Geometry: see drawing. Coordinates: mm, zero at the bounding-box minimum. Coordinates: 2 decimals unless noted, no trailing zeros. Loops run counter-clockwise (first coordinate to the right, second up) from the corner with the lowest first, then second, coordinate; pieces in that order, holes last. Notation, with made-up numbers: (59.25, -32) - (112.25, -32) arc R5 ccw to (112.25, -24) - close; hole circle Ø3 at (22, -35). An arc over 180 degrees is marked (long way). Answer in a Markdown table with one row per item.
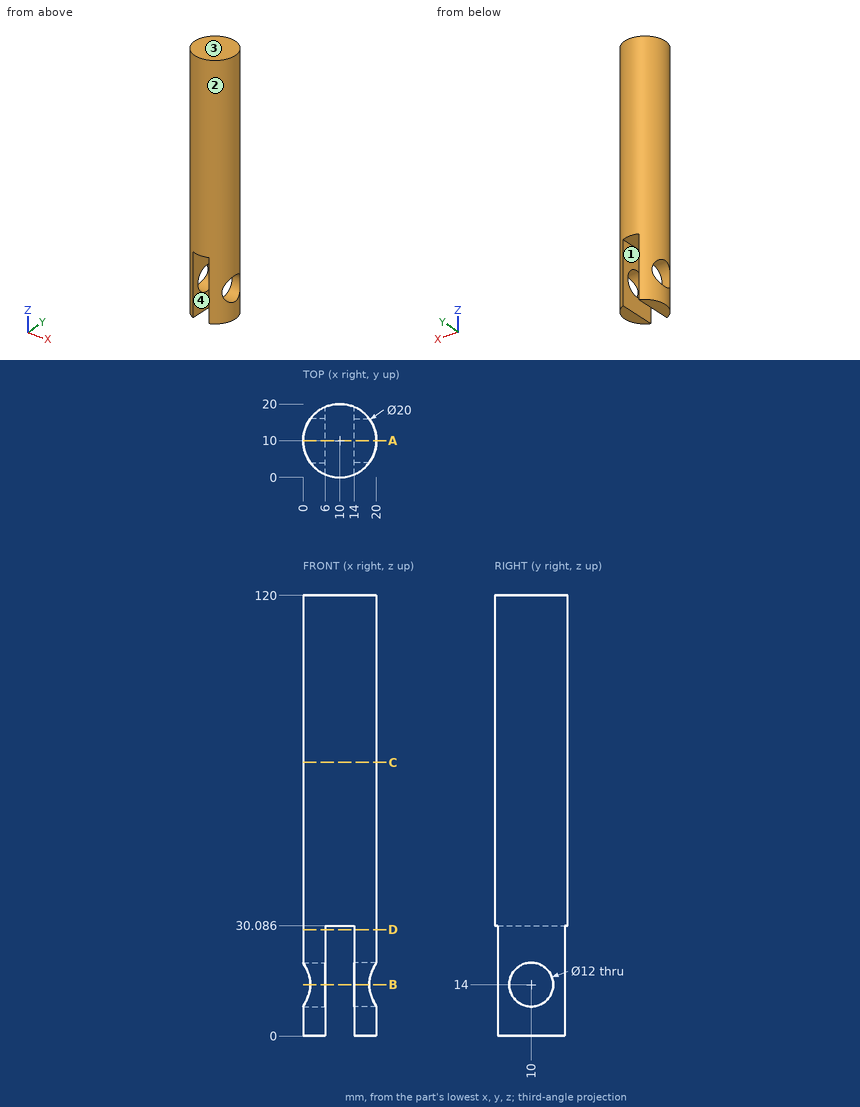
(1) Cut plane A-A on y = 10. Output: boundary loops of the cut face in (x, z).
Verdict:
| item | result |
|---|---|
| outline | (0, 0) - (6, 0) - (6, 8) - (0, 8) - close; (0, 20) - (6, 20) - (6, 30.09) - (14, 30.09) - (14, 20) - (20, 20) - (20, 120) - (0, 120) - close; (14, 0) - (20, 0) - (20, 8) - (14, 8) - close |
(2) First-contact query: pin 1 Ø12 at (x, z) = (3.5, 29.5) entering from -Y; pin 2 Ø1.5 at (y, z) = (17, 45.5) entering from -X; pin 3 Ø9.5 at (y, z) = (10, 14) entering from -X; pin 4 Ø9 at (y, z) = (13.5, 15) entering from +X. Flat tips, straight axial feed; report the tip coordinate or a pass-through.
Verdict:
| item | result |
|---|---|
| pin 1 | stops at y = 0.01 |
| pin 2 | stops at x = 2.19 |
| pin 3 | passes through |
| pin 4 | stops at x = 19.66 |
(3) Pull-direction query (X, two-part tool) for the marked faces 1, 2, 3 and 4; classes: pulls with the +X half, pulls with the -X half, needs draft (parallel to the pull), parting line crosses it, or undercut.
Verdict:
| item | result |
|---|---|
| face 1 | undercut |
| face 2 | parting line crosses it |
| face 3 | needs draft |
| face 4 | undercut |
(4) Cut plane C-C on z = 74.5. Output: boundary loops of the cut face in (x, y), then the cut area to 3 significant figures.
Verdict:
| item | result |
|---|---|
| outline | circle Ø20 at (10, 10) |
| area | 314 mm² |
(5) Ray query, probe 1 along Z at (x, y) = (1.75, 10); probe 2 along Y at (x, z) = (9.5, 46); probe 3 along X at (y, z) = (2, 108.5). Return the intervals inside material, ascending.
Verdict:
| item | result |
|---|---|
| probe 1 | z = 0 to 8, 20 to 120 |
| probe 2 | y = 0.01 to 19.99 |
| probe 3 | x = 4 to 16 |
(6) Cut plane B-B on z = 14. Output: boundary loops of the cut face in (x, y) (1 decimal).
Verdict:
| item | result |
|---|---|
| outline | (2, 4) arc R10 ccw to (6, 0.8) - (6, 4) - close; (2, 16) - (6, 16) - (6, 19.2) arc R10 ccw to start; (14, 0.8) arc R10 ccw to (18, 4) - (14, 4) - close; (14, 16) - (18, 16) arc R10 ccw to (14, 19.2) - close |
(7) Cut plane D-D on z = 29. Output: boundary loops of the cut face in (x, y) (1 decimal).
Verdict:
| item | result |
|---|---|
| outline | (6, 0.8) - (6, 19.2) arc R10 ccw to start; (14, 0.8) arc R10 ccw to (14, 19.2) - close |
